Geometry check sheet. Reference: the model listing, model coordinates, mm. Face numbers are marked on the shaded views. Coordinates: 2 decimals unless noted, no trailing zeros. Loops run counter-clockwise (first coordinate to the right, second up) from the corner with the lowest first, then second, coordinate; pieces in that order, holes last. Notation, with made-up numbers: (55, -3.75) -> (84, -3.75) arc R18 cw to (84, 2.25) -> close; hole circle Ø2 at (50, 2). An arc over 180 degrees is marked (long way). Answer as a JSON object with one key per item and string values.
from build123d import *

# Parameters (mm, degrees)
SKETCH29_R    = 1.5
SKETCH28_R    = 1.3
CHAMFER1_SIZE = 0.2


with BuildPart() as part:
    # Sweep1: sweep along a path in Sketch2
    with BuildLine(Plane.XY) as sweep1_path:
        Line((0, 0), (0, -12))
    # Sketch29 → Sweep1 (sweep)
    with BuildSketch(Plane(origin=(0, 0, 0), x_dir=(1, 0, 0), z_dir=(0, 1, 0))):
        Circle(SKETCH29_R)
    sweep(path=sweep1_path.line)

    # Sweep4: sweep along a path in Sketch7
    with BuildLine(Plane.XY) as sweep4_path:
        Line((0, 0), (0, 0.341807316))
        ThreePointArc((0, 0.341807316), (0.39925091, 1.754801875), (1.47892861, 2.749915424))
        Line((1.47892861, 2.749915424), (2.984841176, 3.513513514))
        ThreePointArc((2.984841176, 3.513513514), (0.783200964, 15.953365261), (-4.287966956, 4.382696005))
        Line((-4.287966956, 4.382696005), (-1.5, 2))
    # Sketch28 → Sweep4 (sweep)
    with BuildSketch(Plane(origin=(0, 0, 0), x_dir=(1, 0, 0), z_dir=(0, 1, 0))):
        Circle(SKETCH28_R)
    sweep(path=sweep4_path.line)

    # Chamfer1
    chamfer1_edges = [part.edges().sort_by_distance(p)[0] for p in [
        (-1.5, 0, 0),
        (-1.5, -12, 0),
    ]]
    chamfer(chamfer1_edges, length=CHAMFER1_SIZE - 0.0001)  # a hair under: the kernel refuses the full size


solid = part.part
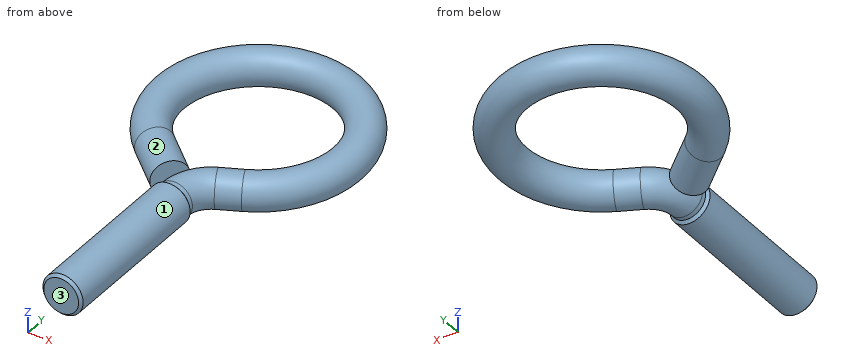
1. Section check A-A, the plane y = -5. Record the boundary of the cut face in (x, z), then the cut area to 3 significant figures.
Evaluation:
{"outline": "circle Ø3 at (0, 0)", "area": "7.07 mm^2"}
2. Thickness scan on probe 1 along X at (y, z) = (3.25, -0.95); probe 2 along Y at (x, z) = (1.75, 0.85); probe 3 along Y at (x, z) = (-3.5, -0.85). Record the ranges inside material, lowest first. Write a range as from..to.
Evaluation:
{"probe 1": "x = -4.33..-1.6, 0.6..4.27", "probe 2": "y = 1.77..3.99, 14.74..16.78", "probe 3": "y = 2.42..5, 13.79..16.13"}
3. Mould release check, pull along X, two halves, no side actions. Record for the marked faces 1, 2 and 3: released by +X, released by -X, zero draft, split by the parting line, or undercut.
Evaluation:
{"face 1": "split by the parting line", "face 2": "undercut", "face 3": "zero draft"}
4. Depth check by flat-ended pin: P1, Ø1, axis at x = 5.5, z = 0, coming from the +Y side; P2, Ø1.5, axis at y = 7.5, z = 0.5, coming from the -X side; P3, Ø2, axis at x = 5.5, y = 13, coming from the +Z side. Enter the tip coordinate at first touch or a pass-through.
Evaluation:
{"P1": "stops at y = 15.52", "P2": "stops at x = -7.79", "P3": "stops at z = 1.3"}
